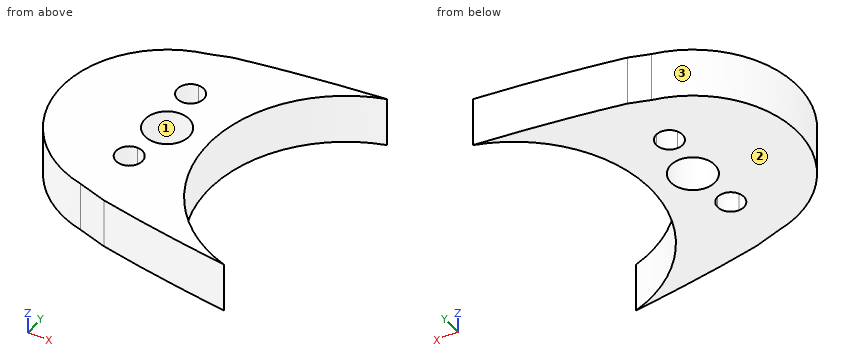
from build123d import *

# Parameters (mm, degrees)
BOSS_EXTRUDE1_START     = 4.25
BOSS_EXTRUDE1_OUTLINE_R = 2.65
BOSS_EXTRUDE1_DEPTH     = 6
CUT_EXTRUDE2_DEPTH      = 49.147003594
CUT_EXTRUDE3_DEPTH      = 46.050777478


# Read off the part's stored shape, not the designer's step: Boss-Extrude1
with BuildPart() as part:
    # Boss-Extrude1 outline → Boss-Extrude1 (new body)
    with BuildSketch(Plane.XY.offset(BOSS_EXTRUDE1_START)):
        with BuildLine():
            ThreePointArc((22.5, 12.599580353), (12.378691282, 0), (22.5, -12.599580353))
            add(Edge.make_bspline(
                [(22.5, -12.599580353), (24.539912926, -13.049943774), (29.005619164, -13.923317691), (36.155474951, -15.030554758), (41.619048326, -15.685620583), (44.644632939, -15.999223801), (45, -16.035396523)],
                knots=[0.544361959, 0.544361959, 0.544361959, 0.544361959, 0.554606397, 0.566671735, 0.579837557, 0.581589368, 0.581589368, 0.581589368, 0.581589368], degree=3))
            ThreePointArc((45, -16.035396523), (30.513983858, 0), (45, 16.035396523))
            add(Edge.make_bspline(
                [(45, 16.035396523), (44.644632939, 15.999223801), (41.619048326, 15.685620583), (36.155474951, 15.030554758), (29.005619164, 13.923317691), (24.539912926, 13.049943774), (22.5, 12.599580353)],
                knots=[0.418410632, 0.418410632, 0.418410632, 0.418410632, 0.420162443, 0.433328265, 0.445393603, 0.455638041, 0.455638041, 0.455638041, 0.455638041], degree=3))
        make_face()
        with Locations((25.281682512, 0)):
            Circle(BOSS_EXTRUDE1_OUTLINE_R, mode=Mode.SUBTRACT)
    extrude(amount=BOSS_EXTRUDE1_DEPTH)

    # Sketch3 → Cut-Extrude2 (cut, through all)
    with BuildSketch(Plane.XY.offset(10.25)):
        with BuildLine():
            ThreePointArc((22.564675294, -12.306634784), (12.678691282, 0), (22.564675294, 12.306634784))
            Line((22.564675294, 12.306634784), (24.936220162, 13.113775399))
            add(Edge.make_bspline(
                [(24.936220162, 13.113775399), (24.122635067, 12.949661044), (23.310473255, 12.77851324), (22.5, 12.599580353)],
                knots=[0.451567846, 0.451567846, 0.451567846, 0.451567846, 0.455638041, 0.455638041, 0.455638041, 0.455638041], degree=3))
            ThreePointArc((22.5, 12.599580353), (12.378691282, 0), (22.5, -12.599580353))
            add(Edge.make_bspline(
                [(22.5, -12.599580353), (23.661751431, -12.856066962), (24.826972348, -13.096557541), (25.994881444, -13.323265839)],
                knots=[0.544361959, 0.544361959, 0.544361959, 0.544361959, 0.550196272, 0.550196272, 0.550196272, 0.550196272], degree=3))
            Line((25.994881444, -13.323265839), (22.564675294, -12.306634784))
        make_face()
        with BuildLine():
            add(Edge.make_bspline(
                [(45, 16.035396523), (44.644632939, 15.999223801), (43.577975433, 15.888664266), (42.511942906, 15.772070236), (41.801329262, 15.691443866)],
                knots=[0.418410632, 0.418410632, 0.418410632, 0.418410632, 0.420162443, 0.423669783, 0.423669783, 0.423669783, 0.423669783], degree=3))
            ThreePointArc((41.801329262, 15.691443866), (30.213983858, 0), (41.801329262, -15.691443866))
            add(Edge.make_bspline(
                [(41.801329262, -15.691443866), (42.511942906, -15.772070236), (43.577975433, -15.888664266), (44.644632939, -15.999223801), (45, -16.035396523)],
                knots=[0.576330217, 0.576330217, 0.576330217, 0.576330217, 0.579837557, 0.581589368, 0.581589368, 0.581589368, 0.581589368], degree=3))
            ThreePointArc((45, -16.035396523), (30.513983858, 0), (45, 16.035396523))
        make_face()
    extrude(amount=-CUT_EXTRUDE2_DEPTH, mode=Mode.SUBTRACT)

    # Sketch4 → Cut-Extrude3 (cut, through all)
    with BuildSketch(Plane.XY.offset(10.25)):
        with BuildLine():
            ThreePointArc((25.993828758, 5.9), (25.532521939, 7.01369318), (24.418828758, 7.475))
            Line((24.418828758, 7.475), (24.418828758, 4.325))
            ThreePointArc((24.418828758, 4.325), (25.532521939, 4.78630682), (25.993828758, 5.9))
        make_face()
        with BuildLine():
            Line((24.418828758, 4.325), (24.418828758, 7.475))
            ThreePointArc((24.418828758, 7.475), (22.843828758, 5.9), (24.418828758, 4.325))
        make_face()
        with BuildLine():
            ThreePointArc((25.993828758, -5.9), (25.532521939, -4.78630682), (24.418828758, -4.325))
            Line((24.418828758, -4.325), (24.418828758, -7.475))
            ThreePointArc((24.418828758, -7.475), (25.532521939, -7.01369318), (25.993828758, -5.9))
        make_face()
        with BuildLine():
            Line((24.418828758, -7.475), (24.418828758, -4.325))
            ThreePointArc((24.418828758, -4.325), (22.843828758, -5.9), (24.418828758, -7.475))
        make_face()
    extrude(amount=-CUT_EXTRUDE3_DEPTH, mode=Mode.SUBTRACT)


solid = part.part
The listing builds one solid part. Answer for the finished solid, in the listing's coordinates (mm). Face numbers are marked on the shaded views. Give positions to 0.01 mm unless a question says otherwise; leave off trailing zeros. Loops run counter-clockwise (first coordinate to the right, second up) from the corner with the lowest first, then second, coordinate; pieces in that order, holes last.
Item 1: A cutting plane is placed at C-C (y = -9.5). Give the vertices of the cut face in (x, z).
Derived:
outline: (17, 4.25) - (33.24, 4.25) - (33.24, 10.25) - (17, 10.25) - close
Item 2: A cutting plane is placed at B-B (z = 8.5). Give the number of separate pieces and of enclosed holes in the cut face, then the cut area to 3 significant figures.
Derived:
separate pieces: 1
enclosed holes: 3
area: 427 mm2
Item 3: A cutting plane is placed at A-A (y = 0). Give the vertices of the cut face in (x, z).
Derived:
outline: (12.68, 4.25) - (22.63, 4.25) - (22.63, 10.25) - (12.68, 10.25) - close; (27.93, 4.25) - (30.21, 4.25) - (30.21, 10.25) - (27.93, 10.25) - close
Item 4: A cutting plane is placed at D-D (x = 17.25). Give the vertices of the cut face in (y, z), then the cut area to 3 significant figures.
Derived:
outline: (-9.71, 4.25) - (9.71, 4.25) - (9.71, 10.25) - (-9.71, 10.25) - close
area: 117 mm2
Item 5: Determine the mould class of the marked faces 1, 2 and 3 for opening direction X: +X half, -X half, draft (parallel to the pull), parting line (faces both ways), or undercut.
Derived:
face 1: undercut
face 2: draft
face 3: -X half
Item 6: Find the intervals of material crossed by line 1 along Y through (x, z) = (23, 8.5); line 2 along Y through (x, z) = (24, 5.75); line 3 along X through (y, z) = (1.5, 8.25), in increasing order.
Derived:
line 1: y = -12.44 to -6.58, -5.22 to -1.35, 1.35 to 5.22, 6.58 to 12.45
line 2: y = -12.73 to -7.42, -4.38 to -2.32, 2.32 to 4.38, 7.42 to 12.8
line 3: x = 12.77 to 23.1, 27.47 to 30.28
Item 7: This flat-tipped pin is pushed along its axis until it touches: pin 1 Ø1.5 at (y, z) = (9.5, 8.5) entering from +X. Where does it stop, or does it pass through?
Derived:
pin 1: stops at x = 33.81
